Build history of the part. All positions in model axes, mm. A direction names the side the tool comes from. Round coordinates to 2 decimals unless told otherwise and drop trailing zeros. Order: outer loops, then holes, each group sorted by start corner. A loop starts at its lowest first (then second) coordinate and runs counter-clockwise, first axis right, second up. Notation, with made-up numbers: (-10.75, 49.5) - (24.25, 49.5) arc R12 ccw to (24.25, 56.5) - close; hole circle Ø3 at (-27.75, -25). An arc over 180 degrees is marked (long way). Write each question's results on one line, items separated by ' | '. Start each with the question number.
```python
from build123d import *

# Parameters (mm, degrees)
BOSS_EXTRUDE1_DEPTH = 15
SKETCH2_W           = 8.404533339
SKETCH2_H           = 40
BOSS_EXTRUDE2_DEPTH = 50
SKETCH3_W           = 20
SKETCH3_H           = 6
CUT_EXTRUDE1_DEPTH  = 2


with BuildPart() as part:
    # Sketch1 → Boss-Extrude1 (new body)
    with BuildSketch(Plane.XY):
        Polygon((21.774193548, 0), (26.564516129, 0), (26.564516129, 47.685483871), (34.838709677, 47.685483871), (34.838709677, 0), (41.806451613, 0), (41.806451613, 25.040322581), (58.5, 25.040322581), (58.5, 0), (60, 0), (60, -40), (0, -40), (0, -13.862903226), (-34.838709677, -13.862903226), (-34.838709677, 0), (-34.838709677, 27.072580645), (-19.306451613, 27.072580645), (-19.306451613, 0), (0, 0), (0, 45.072580645), (8.129032258, 45.072580645), (8.129032258, 0), (13.935483871, 0), (13.935483871, 51.60483871), (21.774193548, 51.60483871), align=None)
    extrude(amount=BOSS_EXTRUDE1_DEPTH)

    # Sketch2 → Boss-Extrude2 (add)
    with BuildSketch(Plane(origin=(0, 0, 0), x_dir=(-1, 0, 0), z_dir=(0, 0, -1))):
        with Locations((-55.797733331, -20)):
            Rectangle(SKETCH2_W, SKETCH2_H)
    extrude(amount=BOSS_EXTRUDE2_DEPTH)

    # Sketch3 → Cut-Extrude1 (cut)
    with BuildSketch(Plane.ZY.offset(-51.595466661)):
        with Locations((-25.300512309, -19.08245708)):
            Rectangle(SKETCH3_W, SKETCH3_H)
    extrude(amount=-CUT_EXTRUDE1_DEPTH, mode=Mode.SUBTRACT)


solid = part.part
```
1. Flat gauge pins, fed straight in: pin 1 Ø16.5 at (x, z) = (-24, 7) entering from -Y; pin 2 Ø2 at (x, z) = (38.5, 11) entering from +Y; pin 3 Ø10 at (x, y) = (-3.5, 3) entering from -Z. Where does each tip first touch, or does it go through?
2. Cut at B-B (z = 5.5). List the corners of the cut face in (x, y), plus the area to 3 significant figures.
3. Cut at A-A (y = 10). List the corners of the cut face in (x, z).
4. Cut at D-D (x = 10). List the corners of the cut face in (y, z).
5. Mould opens along X. For faces 1 (the face through (60, -20, -17)), 2 (the face through (51.595, -25, -25)), 3 (the face through (38, 0, 7)) say: pulls with the +X half, pulls with the -X half, needs draft (parallel to the pull), parting line crosses it, or undercut.
6. 3-axis set-ups, long thin cutter, end or side, ignore diameter. For faces 4 (the face through (-17, -13.863, 7)), 5 (the face through (31, 47.685, 7)), 6 (the face through (-27, 27.073, 7)), 7 (the face through (-19.306, 14, 7)): which of +Z, -Z, +X, -X, +Y, -Y reach the whole face in a straight line?
7. Wall check: line 1 (X direction, y = 12, z = 1.5); line 2 (X direction, y = -26.5, z = -8); line 3 (Y direction, x = 50.5, z = 8.5). Give the ranges that are in metal, low to high. Write a range as from..to.
8. Cut at C-C (y = -30). List the corners of the cut face in (x, z).
A:
1) pin 1: stops at y = -13.86 | pin 2: stops at y = 0 | pin 3: stops at z = 0
2) outline: (-34.84, -13.86) - (0, -13.86) - (0, -40) - (60, -40) - (60, 0) - (58.5, 0) - (58.5, 25.04) - (41.81, 25.04) - (41.81, 0) - (34.84, 0) - (34.84, 47.69) - (26.56, 47.69) - (26.56, 0) - (21.77, 0) - (21.77, 51.6) - (13.94, 51.6) - (13.94, 0) - (8.13, 0) - (8.13, 45.07) - (0, 45.07) - (0, 0) - (-19.31, 0) - (-19.31, 27.07) - (-34.84, 27.07) - close | area: 4,890 mm^2
3) outline: (-34.84, 0) - (-19.31, 0) - (-19.31, 15) - (-34.84, 15) - close; (0, 0) - (8.13, 0) - (8.13, 15) - (0, 15) - close; (13.94, 0) - (21.77, 0) - (21.77, 15) - (13.94, 15) - close; (26.56, 0) - (34.84, 0) - (34.84, 15) - (26.56, 15) - close; (41.81, 0) - (58.5, 0) - (58.5, 15) - (41.81, 15) - close
4) outline: (-40, 0) - (0, 0) - (0, 15) - (-40, 15) - close
5) face 1: pulls with the +X half | face 2: pulls with the -X half | face 3: undercut
6) face 4: +Z, -Z, -X, -Y | face 5: +Z, -Z, +X, +Y | face 6: +Z, -Z, -X, +Y | face 7: +Z, -Z, +Y
7) line 1: x = -34.84..-19.31, 0..8.13, 13.94..21.77, 26.56..34.84, 41.81..58.5 | line 2: x = 51.6..60 | line 3: y = -40..25.04
8) outline: (0, 0) - (51.6, 0) - (51.6, -50) - (60, -50) - (60, 15) - (0, 15) - close
